from build123d import *

# Parameters (mm, degrees)
SKETCH1_W           = 45
SKETCH1_H           = 28
SKETCH1_R           = 1.65
SKETCH1_R_2         = 3.2
SKETCH1_R_3         = 1.75
BOSS_EXTRUDE1_DEPTH = 3
FILLET1_R           = 5


with BuildPart() as part:
    # Sketch1 → Boss-Extrude1 (new body)
    # profile 1 of 2: a face of its own
    with BuildSketch(Plane(origin=(0, 0, 0), x_dir=(1, 0, 0), z_dir=(0, 1, 0))):
        Polygon((-27.5, 14), (-22.5, 14), (22.5, 14), (27.5, 14), (27.5, 22), (-27.5, 22), align=None)
    # profile 2 of 2: a face of its own
    with BuildSketch(Plane(origin=(0, 0, 0), x_dir=(1, 0, 0), z_dir=(0, 1, 0))):
        Rectangle(SKETCH1_W, SKETCH1_H)
        with Locations(Location((19.1, -0.5, 0), (0, 0, 270))):
            Circle(SKETCH1_R, mode=Mode.SUBTRACT)
        with Locations(Location((5.3, -0.5, 0), (0, 0, 270))):
            Circle(SKETCH1_R_2, mode=Mode.SUBTRACT)
        with Locations(Location((-15.3, 8.25, 0), (0, 0, 270))):
            Circle(SKETCH1_R_3, mode=Mode.SUBTRACT)
        with Locations(Location((-15.3, -9.25, 0), (0, 0, 270))):
            Circle(SKETCH1_R_3, mode=Mode.SUBTRACT)
    extrude(amount=BOSS_EXTRUDE1_DEPTH)

    # Fillet1
    fillet1_edges = [part.edges().sort_by_distance(p)[0] for p in [
        (-27.5, 1.5, -22),
        (27.5, 1.5, -22),
        (22.5, 1.5, 14),
        (-22.5, 1.5, 14),
    ]]
    fillet(fillet1_edges, radius=FILLET1_R)


solid = part.part
Here's how the part is built. I have some questions about the finished solid (model axes, mm). A direction names the side the tool comes from. Round coordinates to 2 decimals unless told otherwise and drop trailing zeros. Write each loop counter-clockwise with the first axis right and the second up, starting at its lowest first coordinate (ties: lowest second). Pieces come first, ordered by that corner, then holes. Notation, with made-up numbers: (46.5, 82) -> (56.5, 82) arc R25 cw to (56.5, 103) -> close; hole circle Ø10 at (-4.75, 35.5). An arc over 180 degrees is marked (long way). One line per item, written item: value.
1) We'd pull the mould along X, two halves only. Please class faces 1 (the face through (-16.85, 1.48, 10.06)), 2 (the face through (-26.07, 1.52, -20.5)), 3 (the face through (0, 3, -4)): released by +X, released by -X, zero draft, split by the parting line, or undercut.
Filled sheet:
face 1: undercut
face 2: released by -X
face 3: zero draft
2) For faces 4 (the face through (-22.5, 1, -2)), 5 (the face through (25, 1, -14)), 6 (the face through (-27.5, 1, -16)), which set-ups out of +Z, -Z, +X, -X, +Y, -Y let a thin tool reach every point of the face, with its end or its side?
Filled sheet:
face 4: +Z, -X, +Y, -Y
face 5: +Z, +X, +Y, -Y
face 6: +Z, -Z, -X, +Y, -Y
3) Suppose I cut it at B-B on y = 1.6. List the corners of the cut face in (x, z) for me.
Filled sheet:
outline: (-27.5, -17) arc R5 ccw to (-22.5, -22) -> (22.5, -22) arc R5 ccw to (27.5, -17) -> (27.5, -14) -> (22.5, -14) -> (22.5, 9) arc R5 ccw to (17.5, 14) -> (-17.5, 14) arc R5 ccw to (-22.5, 9) -> (-22.5, -14) -> (-27.5, -14) -> close; hole circle Ø3.5 at (-15.3, -8.25); hole circle Ø3.5 at (-15.3, 9.25); hole circle Ø6.4 at (5.3, 0.5); hole circle Ø3.3 at (19.1, 0.5)
4) Suppose I cut it at A-A on z = -8.25. List the corners of the cut face in (x, y) for me, plus the area to 4 significant figures.
Filled sheet:
outline: (-22.5, 0) -> (-17.05, 0) -> (-17.05, 3) -> (-22.5, 3) -> close; (-13.55, 0) -> (22.5, 0) -> (22.5, 3) -> (-13.55, 3) -> close
area: 124.5 mm2
5) Suppose I cut it at D-D on x = 5.3. List the corners of the cut face in (y, z) for me, plus the area to 3 significant figures.
Filled sheet:
outline: (0, -22) -> (3, -22) -> (3, -2.7) -> (0, -2.7) -> close; (0, 3.7) -> (3, 3.7) -> (3, 14) -> (0, 14) -> close
area: 88.8 mm2
6) Suppose I cut it at C-C on x = -15.3. List the corners of the cut face in (y, z) for me, plus the area to 3 significant figures.
Filled sheet:
outline: (0, -22) -> (3, -22) -> (3, -10) -> (0, -10) -> close; (0, -6.5) -> (3, -6.5) -> (3, 7.5) -> (0, 7.5) -> close; (0, 11) -> (3, 11) -> (3, 14) -> (0, 14) -> close
area: 87.0 mm2
7) If I drill on line 1 (X direction, y = 2.3, z = -8.25); line 2 (X direction, y = 2.1, z = 0.5); line 3 (X direction, y = 2.7, z = -0.5), over which ranges is the centre line in solid material (lowest first)? Write a range as [from, to].
Filled sheet:
line 1: x = [-22.5, -17.05], [-13.55, 22.5]
line 2: x = [-22.5, 2.1], [8.5, 17.45], [20.75, 22.5]
line 3: x = [-22.5, 2.26], [8.34, 17.79], [20.41, 22.5]
8) I'm going to push flat-ended pins straight in: pin 1 Ø0.9 at (x, y) = (-24.5, 1) entering from +Z; pin 2 Ø4 at (x, z) = (19.1, 0.5) entering from +Y; pin 3 Ø1.5 at (y, z) = (2, -1.5) entering from -X. Where does each tip first touch, or does it pass through?
Filled sheet:
pin 1: stops at z = -14
pin 2: stops at y = 3
pin 3: stops at x = -22.5
